Autodesk Inventor part; units mm, degrees
ref_plane "YZ Plane" through (0, 0, 0) normal (1, 0, 0) x (0, 1, 0)
ref_plane "XZ Plane" through (0, 0, 0) normal (0, 1, 0) x (-1, 0, 0)
ref_plane "XY Plane" through (0, 0, 0) normal (0, 0, 1) x (1, 0, 0)
sketch "Sketch1" plane through (0, 0, 0) normal (0, 0, 1) x (1, 0, 0)
  line L0 (0, 0) -> (-145.3374, 0)
  line L1 (-145.3374, 0) -> (-145.3374, -1489.5)
  line L2 (-145.3374, -1489.5) -> (0, -1489.5)
  line L3 (0, -1489.5) -> (0, 0)
  line L4 (-145.3374, -1389.5) -> (-66, -1389.5)
  line L5 (-66, -1389.5) -> (-66, -1384.5)
  line L6 (-66, -1384.5) -> (-145.3374, -1384.5)
  line L7 (-145.3374, -1384.5) -> (-145.3374, -1389.5)
  line L8 (-145.3374, -893) -> (-66, -893)
  line L9 (-66, -893) -> (-66, -888)
  line L10 (-66, -888) -> (-145.3374, -888)
  line L11 (-145.3374, -888) -> (-145.3374, -893)
  line L12 (-145.3374, -396.5) -> (-66, -396.5)
  line L13 (-66, -396.5) -> (-66, -391.5)
  line L14 (-66, -391.5) -> (-145.3374, -391.5)
  line L15 (-145.3374, -391.5) -> (-145.3374, -396.5)
  circle A0 centre (-145.3374, -154.5) radius 30
  point P0 (-145.3374, -391.5)
  point P1 (-145.3374, -1384.5)
  point P2 (-145.3374, -124.5)
  point P3 (-145.3374, -184.5)
  dimension "d0" = 1489.5
  dimension "d1" = 145.3374
  dimension "d2" = 5
  dimension "d4" = 100
  dimension "d7" = 496.5
  dimension "d23" = 66
  dimension "d28" = 60
  dimension "d29" = 1335
extrude "Plate1" add sketch "Sketch1" along normal blind 4 contours L3 L2 L1 L4 L5 L6 L8 L9 L10 L12 L13 L14 A0 L0
sketch "Sketch2" plane through (-4, 0, 0) normal (1, 0, 0) x (0, 1, 0)
  line L0 (-1489.5, 0) -> (0, 0)
  line L1 (0, 0) -> (0, 60)
  line L2 (0, 60) -> (-1489.5, 60)
  line L3 (-1489.5, 60) -> (-1489.5, 0)
edge flange "Flange1" height 60 angle 90 thickness 4 bend radius 4 thickness toward (1, 0, 0) relief tear relief width 4 relief depth 2 edges at (0, -744.75, 4) wall of the first edge with corners at (-4, -1489.5, 0) (-4, 0, 0) (-4, 0, 60) (-4, -1489.5, 60)
bend "Bend1"
corner "Corner1"
chamfer "Corner Chamfer1" distance 3 angle 45 6 edges at (-145.3374, -1389.5, 2) (-145.3374, -1384.5, 2) (-145.3374, -893, 2) (-145.3374, -888, 2) (-145.3374, -391.5, 2) (-145.3374, -396.5, 2)
equation "\"d0\" = Стрингер_длина"
equation "\"d1\" = стрингер_глубина_5"
equation "\"d2\" = паз_под_стрингер_толщина"
equation "\"d7\" = 0.333333 * Стрингер_длина"
equation "\"d23\" = паз_под_стрингер_глубина - Thickness"
equation "\"d28\" = 2 * радиус_выреза_под_сварку"
equation "\"d12\" = Thickness"
equation "\"d13\" = BendReliefWidth"
equation "\"d14\" = BendReliefDepth"
equation "\"d15\" = MinimumRemnant"
equation "\"d16\" = TransitionRadius"
equation "\"d17\" = ребро_усилителей"
equation "\"d19\" = BendRadius"
equation "\"d20\" = CornerReliefSize"
equation "\"d21\" = GapSize"
equation "\"d22\" = JacobiRadiusSize"
equation "\"BendRadius\" = Thickness"
equation "\"BendReliefWidth\" = Thickness"
equation "\"BendReliefDepth\" = 0.5 * Thickness"
equation "\"CornerReliefSize\" = 4 * Thickness"
equation "\"MinimumRemnant\" = 2 * Thickness"
equation "\"TransitionRadius\" = BendRadius"
equation "\"JacobiRadiusSize\" = BendRadius"
equation "\"GapSize\" = Thickness"
properties part number "GBK 0203 stringer 5" material "Steel"
Work out the finished part from the listing and answer in its coordinate system (mm). A direction names the side the tool comes from. Coordinates: 2 decimals unless noted, no trailing zeros. Loops run counter-clockwise (first coordinate to the right, second up) from the corner with the lowest first, then second, coordinate; pieces in that order, holes last. Notation, with made-up numbers: (-21.5, 76.25) -> (18.5, 76.25) arc R8 ccw to (18.5, 84.25) -> close; hole circle Ø2 at (60.5, 65). An arc over 180 degrees is marked (long way). Write each question's results on one line, items separated by ' | '. Start each with the question number.
1) Consider line 1 along Y through (x, z) = (-137, 3); line 2 along X through (y, z) = (-63.5, 33); line 3 along Z through (x, y) = (-9, -330.5). Determine where each line is inside the solid, lowest interval first.
2) Find section B-B on y = -154.5. Determine the outline of the cut face in (x, z).
3) Find section C-C on z = 37. Determine the outline of the cut face in (x, y).
4) Find section D-D on y = -339. Determine the outline of the cut face in (x, z), then the cut area to 3 significant figures.
5) The mould has two halves that part along Y. Classify faces 3 (the flat face through (-51, 0, 3)), 4 (the flat face through (-4, -734, 34)), 5 (the cylindrical face through (-115.345, -153.84, 1.972)), 6 (the flat face through (-51, -1489.5, 3)): pulls with the +Y half, pulls with the -Y half, needs draft (parallel to the pull), parting line crosses it, or undercut.
6) Flat-ended cylindrical pins translate along their axes: P1, Ø2, axis at y = -420.5, z = 44, coming from the -X side; P2, Ø1.2, axis at x = -91, z = 1, coming from the +Y side; P3, Ø1.2, axis at y = -1387.5, z = 2, coming from the -X side; P4, Ø10, axis at x = -98.5, y = -1115.5, coming from the +Z side. Find the tip coordinate at first contact, or state that the pin passes through.
7) For faces 1 (the flat face through (-78, -734, 4)), 2 (the flat face through (-78, -734, 0)), determine the directions among +Z, -Z, +X, -X, +Y, -Y from which every point of the face is accessible in a straight line to the end or side of a thin tool.
8) Find section A-A on x = -87. Determine the outline of the cut face in (y, z).
Response values:
1) line 1: y = -1489.5 to -1389.5, -1384.5 to -893, -888 to -396.5, -391.5 to -183.32, -125.68 to 0 | line 2: x = -4 to 0 | line 3: z = 0 to 4
2) outline: (-115.34, 0) -> (-8, 0) arc R8 ccw to (0, 8) -> (0, 60) -> (-4, 60) -> (-4, 8) arc R4 cw to (-8, 4) -> (-115.34, 4) -> close
3) outline: (-4, -1489.5) -> (0, -1489.5) -> (0, 0) -> (-4, 0) -> close
4) outline: (-145.34, 0) -> (-8, 0) arc R8 ccw to (0, 8) -> (0, 60) -> (-4, 60) -> (-4, 8) arc R4 cw to (-8, 4) -> (-145.34, 4) -> close | area: 795 mm^2
5) face 3: pulls with the +Y half | face 4: needs draft | face 5: undercut | face 6: pulls with the -Y half
6) P1: stops at x = -4 | P2: stops at y = 0 | P3: stops at x = -66 | P4: stops at z = 4
7) face 1: +Z, -X, +Y, -Y | face 2: -Z, +X, -X, +Y, -Y
8) outline: (-1489.5, 0) -> (-1389.5, 0) -> (-1389.5, 4) -> (-1489.5, 4) -> close; (-1384.5, 0) -> (-893, 0) -> (-893, 4) -> (-1384.5, 4) -> close; (-888, 0) -> (-396.5, 0) -> (-396.5, 4) -> (-888, 4) -> close; (-391.5, 0) -> (0, 0) -> (0, 4) -> (-391.5, 4) -> close
